from build123d import *

# Parameters (mm, degrees)
F0_R     = 7.75
F1_DEPTH = 22
F3_DEPTH = 7
F4_R     = 5.9
F5_DEPTH = 13
F6_SIZE  = 1


with BuildPart() as f1:
    # F0 (on Front) → F1 (new body)
    with BuildSketch(Plane.XZ):
        Circle(F0_R)
    extrude(amount=F1_DEPTH)

    # F2 (on face) → F3 (join)
    with BuildSketch(Plane.XZ.offset(22)):
        Polygon((8.5, -4.907477), (8.5, 4.907477), (0, 9.814955), (-8.5, 4.907477), (-8.5, -4.907477), (0, -9.814955), align=None)
    extrude(amount=F3_DEPTH)

    # F4 (on face) → F5 (join)
    with BuildSketch(Plane.XZ.offset(29)):
        Circle(F4_R)
    extrude(amount=F5_DEPTH)

    # F6
    f6_edges = [f1.edges().sort_by_distance(p)[0] for p in [
        (-5.9, -42, 0),
        (-7.75, 0, 0),
    ]]
    chamfer(f6_edges, length=F6_SIZE)


solid = f1.part
Verification items for the finished model (mm, model axes). A direction names the side the tool comes from. Give positions to 0.01 mm unless a question says otherwise; leave off trailing zeros. Order: outer loops, then holes, each group sorted by start corner. A loop starts at its lowest first (then second) coordinate and runs counter-clockwise, first axis right, second up. Notation, with made-up numbers: M 44,-11 L 98,-11 A25 ccw 98,4 Z; hole C 22,52 d6. An arc over 180 degrees is marked long. Answer as a JSON object with one key per item and string values. Group by question number.
1) Cross-section at D-D (y = -35). Enter the section's corners in (x, z).
2) Access from +Z, -Z, +X, -X, +Y, -Y to the whole of each face (thin tool, end or side, straight path). Record for faces 1 (the face through (-1.009, -11.353, 7.684)), 2 (the face through (-5.894, -34.916, 0.259)), 3 (the face through (-8.5, -25, 0)).
3) Cross-section at B-B (y = -25.5). Enter the section's corners in (x, z), then the cut area to 3 significant figures.
4) Scan lines: line 1 along X through (y, z) = (-10.5, -6); line 2 along Y through (x, z) = (7.75, -5.25); line 3 along X through (y, z) = (-39.5, -0.25). Record each from-to range of solid material in increasing order. Write a range as [from, to].
5) Depth check by flat-ended pin: pin 1 Ø1.5 at (y, z) = (-32.5, -3.5) entering from -X; pin 2 Ø4 at (x, y) = (-6, -14.5) entering from -Z; pin 3 Ø3 at (x, y) = (2, -17) entering from -Z. Enter the tip coordinate at first touch or a pass-through.
6) Cross-section at A-A (z = 0). Enter the section's corners in (x, y).
7) Cross-section at C-C (y = -13.5). Enter the section's corners in (x, z), then the cut area to 3 significant figures.
Result sheet:
{
 "1": {"outline": "C 0,0 d11.8"},
 "2": {"face 1": "+Y", "face 2": "-Y", "face 3": "+Z, -Z, -X, +Y, -Y"},
 "3": {"outline": "M -8.5,-4.91 L 0,-9.81 L 8.5,-4.91 L 8.5,4.91 L 0,9.81 L -8.5,4.91 Z", "area": "250 mm2"},
 "4": {"line 1": "x = [-4.91, 4.91]", "line 2": "y = [-29, -22]", "line 3": "x = [-5.89, 5.89]"},
 "5": {"pin 1": "stops at x = -5.22", "pin 2": "stops at z = -6.64", "pin 3": "stops at z = -7.73"},
 "6": {"outline": "M -8.5,-29 L -5.9,-29 L -5.9,-41 L -4.9,-42 L 4.9,-42 L 5.9,-41 L 5.9,-29 L 8.5,-29 L 8.5,-22 L 7.75,-22 L 7.75,-1 L 6.75,0 L -6.75,0 L -7.75,-1 L -7.75,-22 L -8.5,-22 Z"},
 "7": {"outline": "C 0,0 d15.5", "area": "189 mm2"}
}
